Model file for the job. Use its own axes, mm. Face numbers are marked on the shaded views. A direction names the side the tool comes from. Give positions to 0.01 mm unless a question says otherwise; leave off trailing zeros. Write each loop counter-clockwise with the first axis right and the second up, starting at its lowest first coordinate (ties: lowest second). Pieces come first, ordered by that corner, then holes.
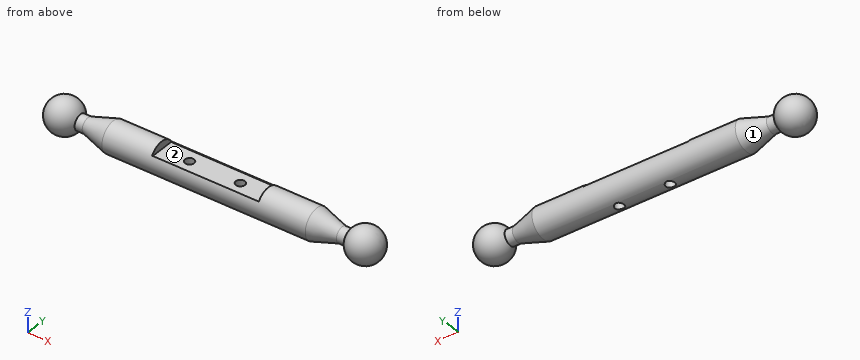
```python
from build123d import *

# Parameters (mm, degrees)
SKETCH4_W          = 210
SKETCH4_H          = 50
CUT_EXTRUDE2_DEPTH = 15
SKETCH5_R          = 9
CUT_EXTRUDE3_DEPTH = 80
DOME1_FACE_RADIUS  = 15
DOME1_HEIGHT       = 65
DOME2_FACE_RADIUS  = 15
DOME2_HEIGHT       = 65


with BuildPart() as part:
    # Sketch2 → Revolve1 (revolve)
    with BuildSketch(Plane.XY):
        Polygon((-265, 0), (265, 0), (265, 15), (250, 15), (200, 30), (-200, 30), (-250, 15), (-265, 15), align=None)
    revolve(axis=Axis((-265, 0, 0), (1, 0, 0)))

    # Sketch4 → Cut-Extrude2 (cut)
    with BuildSketch(Plane.XY.offset(30)):
        Rectangle(SKETCH4_W, SKETCH4_H)
    extrude(amount=-CUT_EXTRUDE2_DEPTH, mode=Mode.SUBTRACT)

    # Sketch5 → Cut-Extrude3 (cut)
    with BuildSketch(Plane.XY.offset(30)):
        with Locations((50, 0)):
            Circle(SKETCH5_R)
        with Locations((-50, 0)):
            Circle(SKETCH5_R)
    extrude(amount=-CUT_EXTRUDE3_DEPTH, mode=Mode.SUBTRACT)

    # Dome1: a dome of height H over a round flat face of radius A is a cap of a sphere of radius (A * A + H * H) / (2 * H)
    dome1_r = (DOME1_FACE_RADIUS * DOME1_FACE_RADIUS + DOME1_HEIGHT * DOME1_HEIGHT) / (2 * DOME1_HEIGHT)
    dome1_base = Plane((265, 0, 0), z_dir=(1, 0, 0))
    with Locations(dome1_base.offset(DOME1_HEIGHT - dome1_r)):
        dome1_ball = Sphere(dome1_r, mode=Mode.PRIVATE)
    add(split(dome1_ball, bisect_by=dome1_base, keep=Keep.TOP, mode=Mode.PRIVATE))

    # Dome2: a dome of height H over a round flat face of radius A is a cap of a sphere of radius (A * A + H * H) / (2 * H)
    dome2_r = (DOME2_FACE_RADIUS * DOME2_FACE_RADIUS + DOME2_HEIGHT * DOME2_HEIGHT) / (2 * DOME2_HEIGHT)
    dome2_base = Plane((-265, 0, 0), z_dir=(-1, 0, 0))
    with Locations(dome2_base.offset(DOME2_HEIGHT - dome2_r)):
        dome2_ball = Sphere(dome2_r, mode=Mode.PRIVATE)
    add(split(dome2_ball, bisect_by=dome2_base, keep=Keep.TOP, mode=Mode.PRIVATE))


solid = part.part
```
1. Pin check, flat tips, straight feed: P1, Ø7.5, axis at y = 6.5, z = 22, coming from the +X side (3 decimals); P2, Ø1.5, axis at x = 196.5, y = 17.5, coming from the -Z side; P3, Ø0.8, axis at x = -15, z = 15.5, coming from the +Y side. Stop position of each tip, or through.
Calculated:
P1: stops at x = 324.115
P2: stops at z = -24.89
P3: stops at y = 25.92
2. Slice it at B-B, the plane x = -50. Write the cut outline in (y, z).
Calculated:
outline: (-25, 15) - (-25, 16.58) arc R30 ccw to (-9, -28.62) - (-9, 15) - close; (9, -28.62) arc R30 ccw to (25, 16.58) - (25, 15) - (9, 15) - close
3. Slice it at A-A, the plane y = 0. Write the cut outline in (x, z), and give its area (3 significant figures).
Calculated:
outline: (-265, -15) - (-250, -15) - (-200, -30) - (-59, -30) - (-59, 15) - (-105, 15) - (-105, 30) - (-200, 30) - (-250, 15) - (-265, 15) arc R34.23 ccw (long way) to start; (-41, -30) - (41, -30) - (41, 15) - (-41, 15) - close; (59, -30) - (200, -30) - (250, -15) - (265, -15) arc R34.23 ccw (long way) to (265, 15) - (250, 15) - (200, 30) - (105, 30) - (105, 15) - (59, 15) - close
area: 31,900 mm2
4. Slice it at D-D, the plane x = -133. Write the cut outline in (y, z), and give its area (3 significant figures).
Calculated:
outline: circle Ø60 at (0, 0)
area: 2,830 mm2
5. Probe probe 1 along Y at (x, z) = (-50, -2); probe 2 along X at (y, z) = (-3.5, -5); probe 3 along X at (y, z) = (7.5, -12). List the from-to ranges inside material, lowest first.
Calculated:
probe 1: y = -29.93 to -9, 9 to 29.93
probe 2: x = -329.45 to -58.29, -41.71 to 41.71, 58.29 to 329.45
probe 3: x = -326.94 to -54.97, -45.03 to 45.03, 54.97 to 326.94
6. Slice it at C-C, the plane z = 0. Write the cut outline in (x, y), and give its area (3 significant figures).
Calculated:
outline: (-265, -15) - (-250, -15) - (-200, -30) - (200, -30) - (250, -15) - (265, -15) arc R34.23 ccw (long way) to (265, 15) - (250, 15) - (200, 30) - (-200, 30) - (-250, 15) - (-265, 15) arc R34.23 ccw (long way) to start; hole circle Ø18 at (-50, 0); hole circle Ø18 at (50, 0)
area: 36,100 mm2
7. Which spindle directions (+Z, -Z, +X, -X, +Y, -Y) get a long thin tool onto all of the face, cutting with end or side? Do the marked faces 1 and 2. Say none if no direction does.
Calculated:
face 1: none
face 2: +Z
